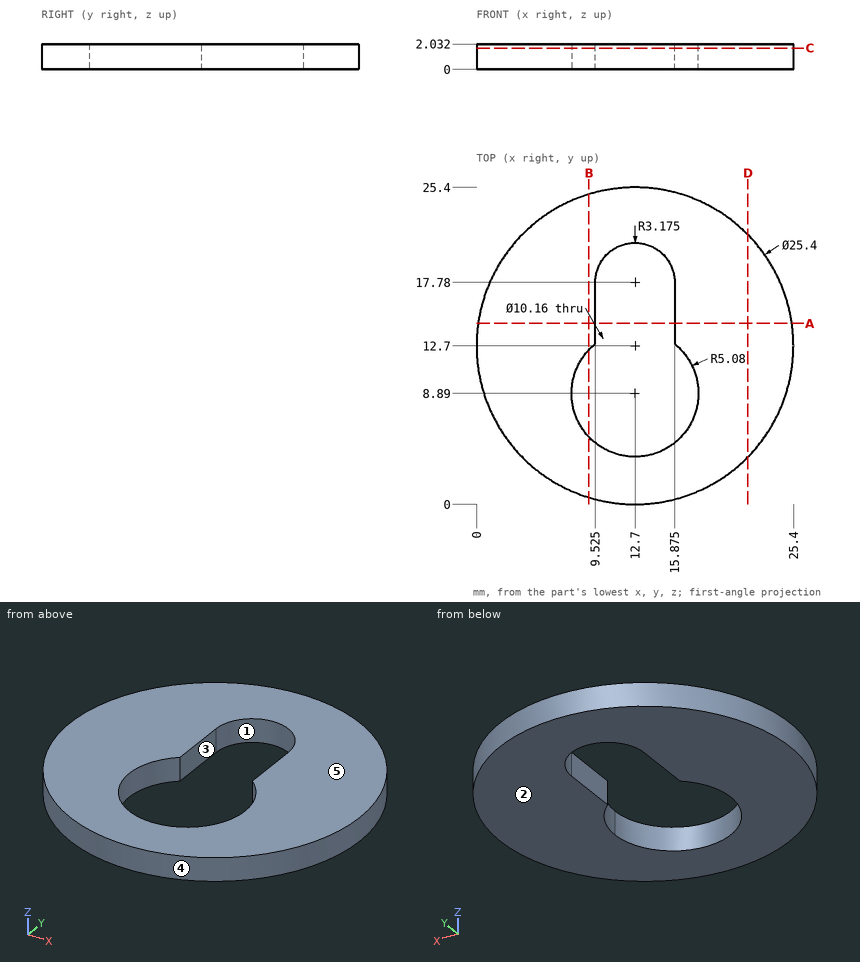
Here's the drawing with two shaded views (mm, measured from the low corner). I have some questions. A direction names the side the tool comes from. Give positions to 0.01 mm unless a question says otherwise; leave off trailing zeros. Write each loop counter-clockwise with the first axis right and the second up, starting at its lowest first coordinate (ties: lowest second). Pieces come first, ordered by that corner, then holes. Notation, with made-up numbers: (83.5, 61) - (131.5, 61) arc R17 ccw to (131.5, 66) - close; hole circle Ø3 at (75, 64.25). An arc over 180 degrees is marked (long way). Write item = value, one per line. Start each with the question number.
1. Thinking about a two-plate mould opening in X: for the marked faces 3, 4 and 5, which applies, released by +X, released by -X, zero draft, split by the parting line, or undercut?
2. Imagine slicing it at C-C (z = 1.7). Please give me the cut outline in (x, y) (3 decimals).
3. Imagine slicing it at D-D (x = 21.75). Please give me the cut outline in (y, z).
4. Imagine slicing it at B-B (x = 9). Please give me the cut outline in (y, z).
5. Imagine slicing it at A-A (y = 14.5). Please give me the cut outline in (x, z) (3 decimals), and give its area (3 significant figures).
6. Please list where these lines run through material, in increasing order: line 1 (Y direction, x = 12.7, z = 0.75) (3 decimals); line 2 (X direction, y = 13.5, z = 1.55) (3 decimals); line 3 (Y direction, x = 10.75, z = 1.1).
7. For pin 1 (3 mm diameter, centred on x = 22.5, y = 4.5, fed in from +Z); pin 2 (0.6 mm diameter, centred on y = 15.5, z = 1, fed in from -X); pin 3 (0.6 mm diameter, centred on y = 14.5, z = 0.5, fed in from +X); pin 4 (1 mm diameter, centred on x = 22.5, z = 1.5, fed in from +Y), each with a flat end and sliding along its axis, tell me the tip position at first contact or that it passes through.
8. On a 3-axis mill with a long thin cutter (end or side, diameter ignored), from which of +Z, -Z, +X, -X, +Y, -Y can I reach the whole of each face in a straight line? I mean the marked faces 1 and 2. Say none if no direction works.
Worked answers:
q1.face_3 = undercut
q1.face_4 = split by the parting line
q1.face_5 = zero draft
q2.outline = circle Ø25.4 at (12.7, 12.7); hole (9.525, 12.856) arc R5.08 ccw (long way) to (15.875, 12.856) - (15.875, 17.78) arc R3.175 ccw to (9.525, 17.78) - close
q3.outline = (3.79, 0) - (21.61, 0) - (21.61, 2.03) - (3.79, 2.03) - close
q4.outline = (0.55, 0) - (5.41, 0) - (5.41, 2.03) - (0.55, 2.03) - close; (12.37, 0) - (24.85, 0) - (24.85, 2.03) - (12.37, 2.03) - close
q5.outline = (0.128, 0) - (9.525, 0) - (9.525, 2.032) - (0.128, 2.032) - close; (15.875, 0) - (25.272, 0) - (25.272, 2.032) - (15.875, 2.032) - close
q5.area = 38.2 mm2
q6.line_1 = 0 to 3.81, 20.955 to 25.4
q6.line_2 = 0.025 to 9.525, 15.875 to 25.375
q6.line_3 = 0.15 to 4.2, 20.29 to 25.25
q7.pin_1 = 2.03
q7.pin_2 = 0.25
q7.pin_3 = 25.31
q7.pin_4 = 21.35
q8.face_1 = +Z, -Z
q8.face_2 = -Z, +X, -X, +Y, -Y
